Could you check a few things on this model? Use its own coordinates, in mm. Coordinates: 2 decimals unless noted, no trailing zeros. Loops run counter-clockwise (first coordinate to the right, second up) from the corner with the lowest first, then second, coordinate; pieces in that order, holes last. Notation, with made-up numbers: M -25,-31 L 33,-31 A24 ccw 33,-6 Z; hole C 8.5,53 d1. An arc over 180 degrees is marked long. Write each question's results on one line, items separated by ' | '.
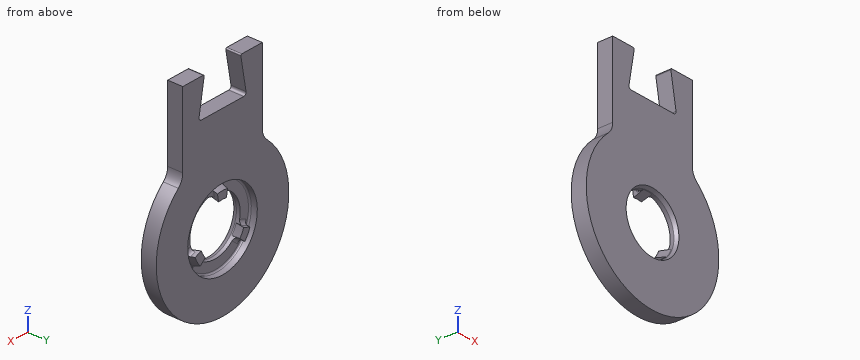
```python
from build123d import *

# Parameters (mm, degrees)
SKETCH1_R           = 4
BOSS_EXTRUDE1_DEPTH = 2
SKETCH2_R           = 10
SKETCH2_R_2         = 3.8
BOSS_EXTRUDE2_DEPTH = 2
SKETCH4_W           = 12
SKETCH4_H           = 0.2
CUT_EXTRUDE1_DEPTH  = 4
FILLET3_R           = 0.35
FILLET4_R           = 0.15
FILLET6_R           = 2
SKETCH13_R          = 5.25
CUT_EXTRUDE5_DEPTH  = 1
REVOLVE2_ANGLE      = 20
CIRPATTERN2_COUNT   = 3
CHAMFER1_SIZE       = 0.5
CHAMFER1_SIZE2      = 0.181985117
FILLET13_R          = 0.5
FILLET14_R          = 0.2


with BuildPart() as part:
    # Sketch1 → Boss-Extrude1 (new body)
    with BuildSketch(Plane(origin=(0, 0, 0), x_dir=(1, 0, 0), z_dir=(0, 1, 0))):
        Polygon((-6, 6), (-6, -13.291502622), (-6, -19), (-2.70227506, -19), (-3.619175359, -13.8), (0, -13.8), (3.619175359, -13.8), (2.70227506, -19), (6, -19), (6, -13.291502622), (6, 6), align=None)
        with Locations(Location((0, 0, 0), (0, 0, 270))):
            Circle(SKETCH1_R, mode=Mode.SUBTRACT)
    extrude(amount=BOSS_EXTRUDE1_DEPTH)

    # Sketch2 → Boss-Extrude2 (add)
    with BuildSketch(Plane(origin=(0, 0, 0), x_dir=(1, 0, 0), z_dir=(0, 1, 0))):
        Circle(SKETCH2_R)
        with Locations(Location((0, 0, 0), (0, 0, 270))):
            Circle(SKETCH2_R_2, mode=Mode.SUBTRACT)
    extrude(amount=BOSS_EXTRUDE2_DEPTH)

    # Sketch4 → Cut-Extrude1 (cut)
    with BuildSketch(Plane(origin=(0, 2, 0), x_dir=(1, 0, 0), z_dir=(0, 1, 0))):
        with Locations((0, -18.9)):
            Rectangle(SKETCH4_W, SKETCH4_H)
    extrude(amount=-CUT_EXTRUDE1_DEPTH, mode=Mode.SUBTRACT)

    # Fillet3
    fillet3_edges = [part.edges().sort_by_distance(p)[0] for p in [
        (3.619175359, 1, 13.8),
        (-3.619175359, 1, 13.8),
    ]]
    fillet(fillet3_edges, radius=FILLET3_R)

    # Fillet4
    fillet4_edges = [part.edges().sort_by_distance(p)[0] for p in [
        (2.737540456, 1, 18.8),
        (-2.737540456, 1, 18.8),
    ]]
    fillet(fillet4_edges, radius=FILLET4_R)

    # Fillet6
    fillet6_edges = [part.edges().sort_by_distance(p)[0] for p in [
        (6, 1, 8),
        (-6, 1, 8),
    ]]
    fillet(fillet6_edges, radius=FILLET6_R)

    # Sketch13 → Cut-Extrude5 (cut)
    with BuildSketch(Plane(origin=(0, 2, 0), x_dir=(1, 0, 0), z_dir=(0, 1, 0))):
        with Locations(Location((0, 0, 0), (0, 0, 270))):
            Circle(SKETCH13_R)
    extrude(amount=-CUT_EXTRUDE5_DEPTH, mode=Mode.SUBTRACT)

    # Sketch12 → Revolve2 (revolve, symmetric)
    with BuildSketch(Plane(origin=(0, 0, 0), x_dir=(0, 0, -1), z_dir=(1, 0, 0))) as revolve2_sk:
        Polygon((-4, 0), (-3.4, 2), (-4.4, 2), (-5, 0), align=None)
    revolve2 = revolve(axis=Axis((0, 0, 0), (0, 1, 0)), revolution_arc=REVOLVE2_ANGLE / 2)
    revolve2 = revolve2 + revolve(revolve2_sk.sketch, axis=Axis((0, 0, 0), (0, -1, 0)), revolution_arc=REVOLVE2_ANGLE / 2)

    # CirPattern2: Revolve2 ×3 about axis
    cirpattern2_axis = Axis((0, 0, 0), (0, 1, 0))
    for i in range(1, CIRPATTERN2_COUNT):
        add(revolve2.rotate(cirpattern2_axis, i * 360 / CIRPATTERN2_COUNT))

    # Chamfer1
    chamfer1_edges = [part.edges().sort_by_distance(p)[0] for p in [
        (0, 0, -3.8),
    ]]
    chamfer1_side = [part.faces().sort_by_distance(p)[0] for p in [
        (0, 0.5, -3.8),
    ]]
    chamfer(chamfer1_edges, length=CHAMFER1_SIZE, length2=CHAMFER1_SIZE2, reference=chamfer1_side[0])

    # Fillet13
    fillet13_edges = [part.edges().sort_by_distance(p)[0] for p in [
        (-0.738004755, 1, 4.18543295),
        (0.738004755, 1, 4.18543295),
        (-3.255688883, 1, -2.731847341),
        (-3.993693638, 1, -1.453585609),
        (3.993693638, 1, -1.453585609),
        (3.255688883, 1, -2.731847341),
    ]]
    fillet(fillet13_edges, radius=FILLET13_R)

    # Fillet14
    fillet14_edges = [part.edges().sort_by_distance(p)[0] for p in [
        (0, 1, -5.25),
        (-4.070319398, 1, -2.35),
        (4.070319398, 1, -2.35),
        (0, 1, 4.7),
    ]]
    fillet(fillet14_edges, radius=FILLET14_R)


solid = part.part
```
(1) Imagine slicing it at A-A, the plane x = 0. List the corners of the cut face in (y, z) for me.
Reported:
outline: M 0,-10 L 2,-10 L 2,-5.25 L 1.2,-5.25 A0.2 cw 1,-5.05 L 1,-3.8 L 0.5,-3.8 L 0,-3.98 Z; M 0,3.98 L 0.5,3.8 L 0.67,3.8 L 2,3.4 L 2,4.4 L 1.14,4.66 A0.2 cw 1,4.85 L 1,5.05 A0.2 cw 1.2,5.25 L 2,5.25 L 2,13.8 L 0,13.8 Z
(2) Will these pins go through, and if not, where does the flat tip stop? P1, Ø10, axis at x = 0, z = 0, coming from the +Y side; P2, Ø0.6, axis at y = 1.5, z = 12.5, coming from the -X side; P3, Ø3, axis at x = 0, z = -1, coming from the +Y side.
Reported:
P1: stops at y = 2 | P2: stops at x = -6 | P3: passes through
(3) Imagine slicing it at D-D, the plane z = 14.75. List the corners of the cut face in (x, y) for me.
Reported:
outline: M -6,0 L -3.45,0 L -3.45,2 L -6,2 Z; M 3.45,0 L 6,0 L 6,2 L 3.45,2 Z
(4) Imagine slicing it at C-C, the plane z = -8. List the corners of the cut face in (x, y) for me, and give its area (3 significant figures).
Reported:
outline: M -6,0 L 6,0 L 6,2 L -6,2 Z | area: 24.0 mm2
(5) Please list where these lines run through material, in increasing order: probe 1 along X at (y, z) = (1.65, 0); probe 2 along X at (y, z) = (0.85, 0); probe 3 along Z at (x, y) = (0, 0.95) (3 decimals). Write a range as from..to.
Reported:
probe 1: x = -10..-5.25, 5.25..10 | probe 2: x = -10..-3.8, 3.8..10 | probe 3: z = -10..-3.8, 3.715..13.8
(6) Imagine slicing it at B-B, the plane z = 0. List the corners of the cut face in (x, y) for me, and give its area (3 significant figures).
Reported:
outline: M -10,0 L -3.98,0 L -3.8,0.5 L -3.8,1 L -5.05,1 A0.2 cw -5.25,1.2 L -5.25,2 L -10,2 Z; M 3.8,0.5 L 3.98,0 L 10,0 L 10,2 L 5.25,2 L 5.25,1.2 A0.2 cw 5.05,1 L 3.8,1 Z | area: 21.8 mm2
